from build123d import *

# Parameters (mm, degrees)
F1_DEPTH  = 280
F2_W      = 60
F2_H      = 338
F3_DEPTH  = 10.001
F5_DEPTH  = 10.001
F6_R      = 8.25
F7_DEPTH  = 10.001
F8_R      = 4.25
F9_DEPTH  = 10.001
F10_W     = 10
F10_H     = 85
F11_DEPTH = 85
F14_DEPTH = 220.001
F15_DEPTH = 280.001


with BuildPart() as f1:
    # F0 (on Right) → F1 (new body)
    with BuildSketch(Plane.YZ):
        Polygon((10, -145), (10, 135), (0, 135), (0, -135), (-338, -135), (-338, -145), align=None)
    extrude(amount=F1_DEPTH)

    # F2 (on face) → F3 (cut, through all)
    with BuildSketch(Plane.XY.offset(-135)):
        with Locations((30, -169)):
            Rectangle(F2_W, F2_H)
    extrude(amount=-F3_DEPTH, mode=Mode.SUBTRACT)

    # F4 (on face) → F5 (cut, through all)
    with BuildSketch(Plane.XZ):
        Polygon((60, -135), (0, -50), (0, -145), (60, -145), align=None)
    extrude(amount=-F5_DEPTH, mode=Mode.SUBTRACT)

    # F6 (on face) → F7 (cut, through all)
    with BuildSketch(Plane.XZ):
        with Locations((30, 104)):
            Circle(F6_R)
        with Locations((255, 104)):
            Circle(F6_R)
        with Locations((255, -14)):
            Circle(F6_R)
        with Locations((30, -14)):
            Circle(F6_R)
    extrude(amount=-F7_DEPTH, mode=Mode.SUBTRACT)

    # F8 (on face) → F9 (cut, through all)
    with BuildSketch(Plane.XY.offset(-135)):
        with Locations((80, -10)):
            Circle(F8_R)
        with Locations((260, -10)):
            Circle(F8_R)
        with Locations((80, -318)):
            Circle(F8_R)
        with Locations((260, -318)):
            Circle(F8_R)
    extrude(amount=-F9_DEPTH, mode=Mode.SUBTRACT)

    # F10 (on face) → F11 (join)
    with BuildSketch(Plane.XZ):
        with Locations((65, -92.5)):
            Rectangle(F10_W, F10_H)
        with Locations((275, -92.5)):
            Rectangle(F10_W, F10_H)
    extrude(amount=F11_DEPTH)

    # F13 (on face) → F14 (cut, through all)
    with BuildSketch(Plane(origin=(60, 0, 0), x_dir=(0, -1, 0), z_dir=(-1, 0, 0))):
        Polygon((85, -50), (0, -50), (85, -135), align=None)
    extrude(amount=-F14_DEPTH, mode=Mode.SUBTRACT)

    # F12 (on face) → F15 (cut, through all)
    with BuildSketch(Plane.YZ.offset(280)):
        Polygon((-85, -135), (0, -50), (-85, -50), align=None)
    extrude(amount=-F15_DEPTH, mode=Mode.SUBTRACT)


solid = f1.part
Read the model definition and answer for the solid it produces. Units are mm, in the model's axes. A direction names the side the tool comes from. Coordinates: 2 decimals unless noted, no trailing zeros. Order: outer loops, then holes, each group sorted by start corner. A loop starts at its lowest first (then second) coordinate and runs counter-clockwise, first axis right, second up. Notation, with made-up numbers: M 69,21 L 74,21 A20 cw 74,44 Z; hole C -32,-36 d2. An arc over 180 degrees is marked long. Put each result on its own line as item: value. Start each with the question number.
Item 1: Given pin 1 Ø7.5 at (x, y) = (260, -10) entering from -Z; pin 2 Ø10 at (x, y) = (136.5, -86) entering from +Z; pin 3 Ø19 at (x, z) = (255, 104) entering from -Y, each flat-ended and moving along its own axis, determine where each tip first touches the part or whether it passes through.
Item 2: Consider probe 1 along Z at (x, y) = (30, 4); probe 2 along Z at (x, y) = (192.5, -32.5); probe 3 along Y at (x, z) = (200, 12). Determine where each line is inside the solid, lowest interval first. Write a range as [from, to].
Item 3: Section D-D, the plane x = 202.5 is taken. Determine the outline of the cut face in (y, z).
Item 4: Section B-B, the plane z = 104 is taken. Determine the outline of the cut face in (x, y), plus the area to 3 significant figures.
Item 5: Section C-C, the plane x = 80 is taken. Determine the outline of the cut face in (y, z), plus the area to 3 significant figures.
Item 6: Section A-A, the plane y = -10 is taken. Determine the outline of the cut face in (x, z), plus the area to 3 significant figures.
Item 7: The mould has two halves that part along Y. Classify faces 3 (the face through (70, -32, -103)), 4 (the face through (65, -42, -92)), 5 (the face through (255.754, -9.813, -139.93)): +Y half, -Y half, draft (parallel to the pull), parting line (faces both ways), or undercut.
Item 8: For faces 1 (the face through (270, -32, -103)), 2 (the face through (21.758, 4.93, -13.637)), determine the directions among +Z, -Z, +X, -X, +Y, -Y from which every point of the face is accessible in a straight line to the end or side of a thin tool.
Computed:
1. pin 1: passes through
1. pin 2: stops at z = -135
1. pin 3: stops at y = 0
2. probe 1: z = [-92.5, -22.25], [-5.75, 95.75], [112.25, 135]
2. probe 2: z = [-145, -135]
2. probe 3: y = [0, 10]
3. outline: M -338,-145 L 10,-145 L 10,135 L 0,135 L 0,-135 L -338,-135 Z
4. outline: M 0,0 L 21.75,0 L 21.75,10 L 0,10 Z; M 38.25,0 L 246.75,0 L 246.75,10 L 38.25,10 Z; M 263.25,0 L 280,0 L 280,10 L 263.25,10 Z
4. area: 2,470 mm2
5. outline: M -338,-145 L -322.25,-145 L -322.25,-135 L -338,-135 Z; M -313.75,-145 L -14.25,-145 L -14.25,-135 L -313.75,-135 Z; M -5.75,-145 L 10,-145 L 10,135 L 0,135 L 0,-135 L -5.75,-135 Z
5. area: 6,010 mm2
6. outline: M 60,-145 L 75.75,-145 L 75.75,-135 L 70,-135 L 70,-60 L 60,-60 Z; M 84.25,-145 L 255.75,-145 L 255.75,-135 L 84.25,-135 Z; M 264.25,-145 L 280,-145 L 280,-60 L 270,-60 L 270,-135 L 264.25,-135 Z
6. area: 3,530 mm2
7. face 3: draft
7. face 4: -Y half
7. face 5: undercut
8. face 1: +Z, -Y
8. face 2: +Y, -Y
